Check sheet for the drawn part. Datum: minimum x, y, z corner. Units: mm. A direction names the side the tool comes from. Give positions to 0.01 mm unless a question says otherwise; leave off trailing zeros. Order: outer loops, then holes, each group sorted by start corner. A loop starts at its lowest first (then second) coordinate and runs counter-clockwise, first axis right, second up.
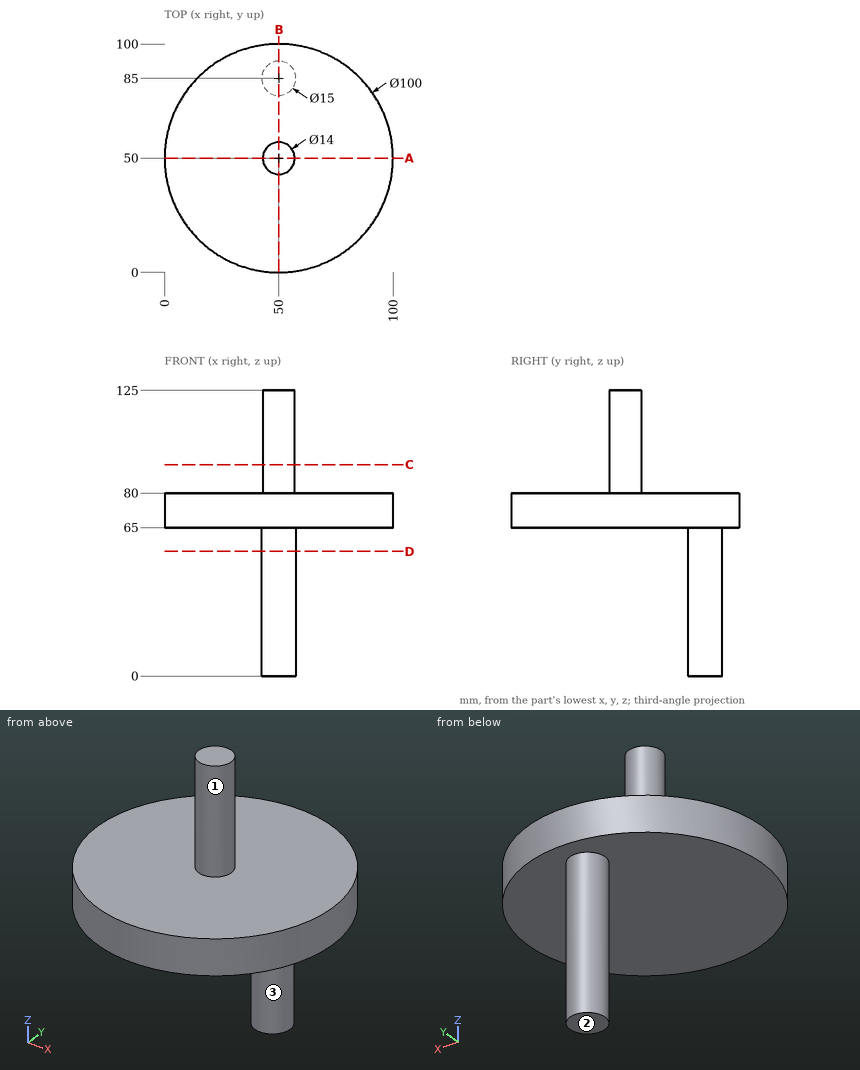
Item 1: Sectioned sample at C-C (z = 92.5). Enter the section's corners in (x, y), and give its area (3 significant figures).
Reported:
outline: circle Ø14 at (50, 50)
area: 154 mm2
Item 2: Sectioned sample at B-B (x = 50). Enter the section's corners in (y, z), and give its area (4 significant figures).
Reported:
outline: (0, 65) - (77.5, 65) - (77.5, 0) - (92.5, 0) - (92.5, 65) - (100, 65) - (100, 80) - (57, 80) - (57, 125) - (43, 125) - (43, 80) - (0, 80) - close
area: 3,105 mm2
Item 3: Sectioned sample at A-A (y = 50). Enter the section's corners in (x, z).
Reported:
outline: (0, 65) - (100, 65) - (100, 80) - (57, 80) - (57, 125) - (43, 125) - (43, 80) - (0, 80) - close
Item 4: Set-up check for the marked faces 1, 2 and 3: record each of +Z, -Z, +X, -X, +Y, -Y from which the full face is reachable in a straight line by a thin tool's end or side.
Reported:
face 1: +Z
face 2: -Z, +X, -X, +Y, -Y
face 3: -Z
Item 5: Scan lines: L1, parallel to Z at x = 83.5, y = 37.5; L2, parallel to X at y = 85.5, z = 30.5; L3, parallel to X at y = 84, z = 69. Record each from-to range of solid material in increasing order.
Reported:
L1: z = 65 to 80
L2: x = 42.52 to 57.48
L3: x = 13.34 to 86.66
Item 6: Sectioned sample at D-D (z = 54.5). Enter the section's corners in (x, y), and give its area (3 significant figures).
Reported:
outline: circle Ø15 at (50, 85)
area: 177 mm2
Item 7: Gauge pin test, flat ends, axial feed: pin 1 (5 mm diameter, centred on y = 87.5, z = 36.5, fed in from -X); pin 2 (10 mm diameter, centred on y = 58, z = 102, fed in from +X); pin 3 (3 mm diameter, centred on y = 24, z = 76.5, fed in from -X). Record the tip position at first contact, or that the pin passes through.
Reported:
pin 1: stops at x = 42.5
pin 2: stops at x = 56.32
pin 3: stops at x = 6.41
